Design review of the part built by this model. Coordinates are the model's own, in mm. A direction names the side the tool comes from. Coordinates: 2 decimals unless noted, no trailing zeros. Write each loop counter-clockwise with the first axis right and the second up, starting at its lowest first coordinate (ties: lowest second). Pieces come first, ordered by that corner, then holes. Notation, with made-up numbers: (50.5, -8.75) - (104.5, -8.75) arc R17 cw to (104.5, -3.75) - close; hole circle Ø7 at (9.5, -22). An arc over 180 degrees is marked (long way). Answer as CSV lines item,"result". Start each with the question number.
Q1. Mouldability with a two-part tool opening along Y and no side actions: class faces 4 (the face through (14.206, 15.557, 32.028)), 5 (the face through (0, 0, 46)), 6 (the face through (-19.421, 19.503, 16.762)) as pulls with the +Y half, pulls with the -Y half, needs draft (parallel to the pull), parting line crosses it, or undercut.
Q2. Machinability: for faces 1 (the face through (-16, 16, 30)), 2 (the face through (-24, 0, 6)), 3 (the face through (-24, 0, 7.5)), which of the approach directions +Z, -Z, +X, -X, +Y, -Y give a long, thin tool a straight path to every point of the face, cutting with its end or side? Answer none if there is none.
Q3. We need section B-B (x = -23). Write out the cut boundary in (y, z), plus the area to 3 significant figures.
Q4. We need section C-C (y = 0). Write out the cut boundary in (x, z).
Q5. We need section D-D (z = 19.5). Write out the cut boundary in (x, y), plus the area to 3 significant figures.
Q6. For line 1 along Y through (x, z) = (0, 35.3); line 2 along Y through (x, z) = (15.5, 32.7) (3 decimals); line 3 along X through (y, z) = (15, 32), list the stretches that pass through material, from the lowest coordinate up. Write a range as [from, to].
Q7. We need section A-A (z = 28). Write out the cut boundary in (x, y), plus the area to 3 significant figures.
Q8. Clearance check with flat-ended pins moving along their axes: pin 1 (1.2 mm diameter, centred on x = -25, y = -0.5, fed in from +Z); pin 2 (12 mm diameter, centred on y = 13, z = 25.5, fed in from -X); pin 3 (2 mm diameter, centred on x = -10, y = -6.5, fed in from +Z). State where each tip first meets the part, or that it passes through.
from build123d import *

# Parameters (mm, degrees)
PAD007_DEPTH    = 4
SKETCH010_W     = 16
SKETCH010_H     = 8
PAD006_DEPTH    = 1
SKETCH008_R     = 2.5
PAD004_DEPTH    = 19
SKETCH006_R     = 11
PAD003_DEPTH    = 2
SKETCH007_R     = 9
POCKET003_DEPTH = 2
PAD002_DEPTH    = 7.5
SKETCH003_R     = 9
POCKET_DEPTH    = 1
SKETCH004_R     = 4.25
POCKET001_DEPTH = 6
SKETCH005_R     = 1.295
POCKET002_DEPTH = 4
PAD001_DEPTH    = 17
PAD_DEPTH       = 9.5


with BuildPart() as pad007:
    # Sketch011 → Pad007 (new body)
    with BuildSketch(Plane.YZ.offset(-22)):
        with BuildLine():
            Line((2.5, 7.5), (-2.5, 7.5))
            ThreePointArc((-2.5, 7.5), (-2.853553, 7.353553), (-3, 7))
            Line((-3, 7), (-3, 6.5))
            ThreePointArc((-3, 6.5), (-2.853553, 6.146447), (-2.5, 6))
            Line((-2.5, 6), (2.5, 6))
            ThreePointArc((2.5, 6), (2.853553, 6.146447), (3, 6.5))
            Line((3, 6.5), (3, 7))
            ThreePointArc((3, 7), (2.853553, 7.353553), (2.5, 7.5))
        make_face()
    extrude(amount=-PAD007_DEPTH)


with BuildPart() as pad006:
    # Sketch010 → Pad006 (new body)
    with BuildSketch(Plane.YZ.offset(-21)):
        with Locations((0, 5.5)):
            Rectangle(SKETCH010_W, SKETCH010_H)
    extrude(amount=-PAD006_DEPTH)


with BuildPart() as pad004:
    # Sketch008 → Pad004 (new body)
    with BuildSketch(Plane.XY.offset(27)):
        Circle(SKETCH008_R)
    extrude(amount=PAD004_DEPTH)


with BuildPart() as fusion001:
    # Sketch006 → Pad003 (new body)
    with BuildSketch(Plane.XY.offset(34)):
        Circle(SKETCH006_R)
    extrude(amount=PAD003_DEPTH)

    # Sketch007 → Pocket003 (cut)
    with BuildSketch(Plane.XY.offset(36)):
        Circle(SKETCH007_R)
    extrude(amount=-POCKET003_DEPTH, mode=Mode.SUBTRACT)

    # Fusion001: union Pad004
    add(pad004.part)


with BuildPart() as f_6mm:
    # Sketch002 → Pad002 (new body)
    with BuildSketch(Plane.XY.offset(26.5)):
        with BuildLine():
            Line((-15.75, 21), (15.75, 21))
            ThreePointArc((21, 15.75), (19.462311, 19.462311), (15.75, 21))
            Line((21, 15.75), (21, -15.75))
            ThreePointArc((15.75, -21), (19.462311, -19.462311), (21, -15.75))
            Line((15.75, -21), (-15.75, -21))
            ThreePointArc((-21, -15.75), (-19.462311, -19.462311), (-15.75, -21))
            Line((-21, -15.75), (-21, 15.75))
            ThreePointArc((-15.75, 21), (-19.462311, 19.462311), (-21, 15.75))
        make_face()
    extrude(amount=PAD002_DEPTH)

    # Sketch003 → Pocket (cut)
    with BuildSketch(Plane.XY.offset(34)):
        Circle(SKETCH003_R)
    extrude(amount=-POCKET_DEPTH, mode=Mode.SUBTRACT)

    # Sketch004 → Pocket001 (cut)
    with BuildSketch(Plane.XY.offset(33)):
        Circle(SKETCH004_R)
    extrude(amount=-POCKET001_DEPTH, mode=Mode.SUBTRACT)


with BuildPart() as m3:
    add(f_6mm.part)

    # Sketch005 → Pocket002 (cut)
    with BuildSketch(Plane.XY.offset(34)):
        with Locations((15.5, 15.5)):
            Circle(SKETCH005_R)
        with Locations((-15.5, 15.5)):
            Circle(SKETCH005_R)
        with Locations((-15.5, -15.5)):
            Circle(SKETCH005_R)
        with Locations((15.5, -15.5)):
            Circle(SKETCH005_R)
    extrude(amount=-POCKET002_DEPTH, mode=Mode.SUBTRACT)


with BuildPart() as fusion002:
    add(f_6mm.part)

    add(m3.part, mode=Mode.INTERSECT)

    # Fusion002: union Fusion001
    add(fusion001.part)


with BuildPart() as pad001:
    # Sketch001 → Pad001 (new body)
    with BuildSketch(Plane.XY.offset(9.5)):
        with BuildLine():
            Line((-15.75, 21), (15.75, 21))
            ThreePointArc((21, 15.75), (19.462311, 19.462311), (15.75, 21))
            Line((21, 15.75), (21, -15.75))
            ThreePointArc((15.75, -21), (19.462311, -19.462311), (21, -15.75))
            Line((15.75, -21), (-15.75, -21))
            ThreePointArc((-21, -15.75), (-19.462311, -19.462311), (-15.75, -21))
            Line((-21, -15.75), (-21, 15.75))
            ThreePointArc((-15.75, 21), (-19.462311, 19.462311), (-21, 15.75))
        make_face()
    extrude(amount=PAD001_DEPTH)


with BuildPart() as fusion005:
    # Sketch → Pad (new body)
    with BuildSketch(Plane.XY):
        with BuildLine():
            Line((-15.75, 21), (15.75, 21))
            ThreePointArc((21, 15.75), (19.462311, 19.462311), (15.75, 21))
            Line((21, 15.75), (21, -15.75))
            ThreePointArc((15.75, -21), (19.462311, -19.462311), (21, -15.75))
            Line((15.75, -21), (-15.75, -21))
            ThreePointArc((-21, -15.75), (-19.462311, -19.462311), (-15.75, -21))
            Line((-21, -15.75), (-21, 15.75))
            ThreePointArc((-15.75, 21), (-19.462311, 19.462311), (-21, 15.75))
        make_face()
    extrude(amount=PAD_DEPTH)

    # Fusion: union Pad001
    add(pad001.part)

    # Fusion003: union Fusion002
    add(fusion002.part)

    # Fusion004: union Pad006
    add(pad006.part)

    # Fusion005: union Pad007
    add(pad007.part)


solid = fusion005.part
Results list:
1,face 4,"undercut"
1,face 5,"needs draft"
1,face 6,"pulls with the +Y half"
2,face 1,"+Z"
2,face 2,"-Z, -X, +Y, -Y"
2,face 3,"+Z, -X, +Y, -Y"
3,outline,"(-3, 6.5) arc R0.5 ccw to (-2.5, 6) - (2.5, 6) arc R0.5 ccw to (3, 6.5) - (3, 7) arc R0.5 ccw to (2.5, 7.5) - (-2.5, 7.5) arc R0.5 ccw to (-3, 7) - close"
3,area,"8.79 mm2"
4,outline,"(-26, 6) - (-22, 6) - (-22, 1.5) - (-21, 1.5) - (-21, 0) - (21, 0) - (21, 34) - (11, 34) - (11, 36) - (9, 36) - (9, 33) - (4.25, 33) - (4.25, 27) - (2.5, 27) - (2.5, 46) - (-2.5, 46) - (-2.5, 27) - (-4.25, 27) - (-4.25, 33) - (-9, 33) - (-9, 36) - (-11, 36) - (-11, 34) - (-21, 34) - (-21, 9.5) - (-22, 9.5) - (-22, 7.5) - (-26, 7.5) - close"
5,outline,"(-21, -15.75) arc R5.25 ccw to (-15.75, -21) - (15.75, -21) arc R5.25 ccw to (21, -15.75) - (21, 15.75) arc R5.25 ccw to (15.75, 21) - (-15.75, 21) arc R5.25 ccw to (-21, 15.75) - close"
5,area,"1,740 mm2"
6,line 1,"y = [-11, -9], [-2.5, 2.5], [9, 11]"
6,line 2,"y = [-21, -16.795], [-14.205, 14.205], [16.795, 21]"
6,line 3,"x = [-21, -16.69], [-14.31, 14.31], [16.69, 21]"
7,outline,"(-21, -15.75) arc R5.25 ccw to (-15.75, -21) - (15.75, -21) arc R5.25 ccw to (21, -15.75) - (21, 15.75) arc R5.25 ccw to (15.75, 21) - (-15.75, 21) arc R5.25 ccw to (-21, 15.75) - close; circle Ø5 at (0, 0); hole circle Ø8.5 at (0, 0)"
7,area,"1,700 mm2"
8,pin 1,"stops at z = 7.5"
8,pin 2,"stops at x = -21"
8,pin 3,"stops at z = 36"
